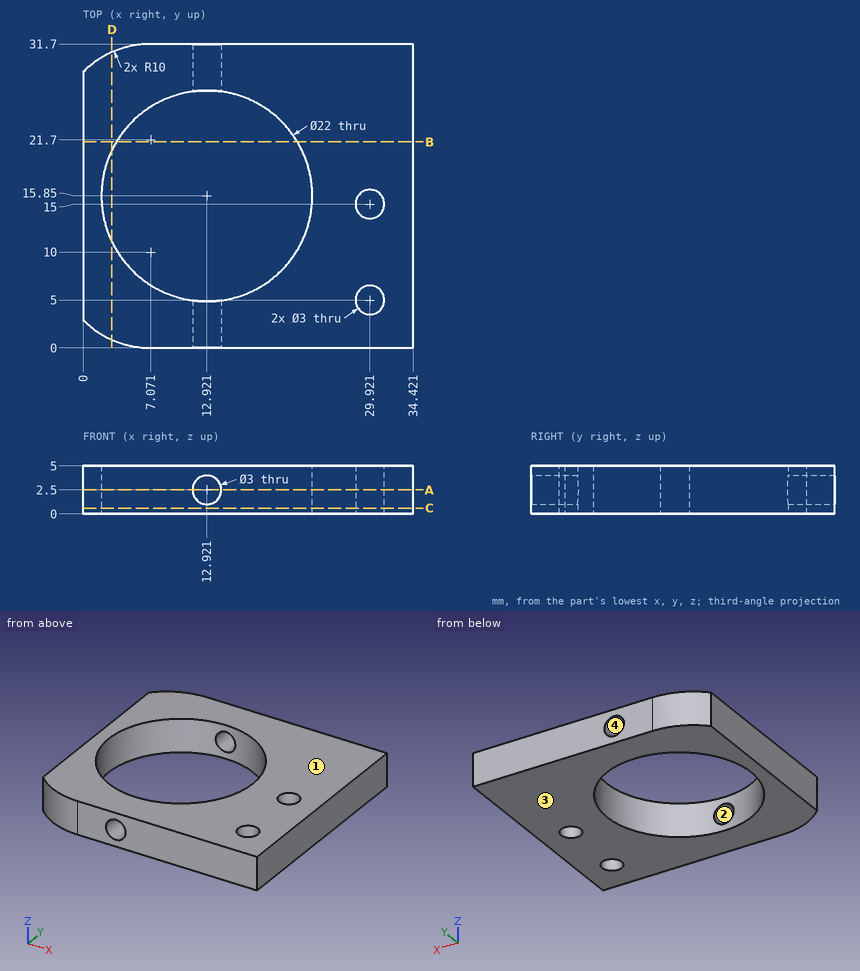
Input: dimensioned drawing with shaded views. Units: mm. Origin: part minimum x, y, z. Round coordinates to 2 decimals unless told otherwise and drop trailing zeros. Order: outer loops, then holes, each group sorted by start corner. A loop starts at its lowest first (then second) coordinate and runs counter-clockwise, first axis right, second up.
1. Cut plane D-D, the plane x = 3. Output: boundary loops of the cut face in (y, z), then the cut area to 3 significant figures.
The answers:
outline: (0.87, 0) - (11.1, 0) - (11.1, 5) - (0.87, 5) - close; (20.6, 0) - (30.83, 0) - (30.83, 5) - (20.6, 5) - close
area: 102 mm2
2. Cut plane A-A, the plane z = 2.5. Output: boundary loops of the cut face in (x, y), then the cut area to 3 significant figures.
The answers:
outline: (0, 2.93) arc R10 ccw to (7.07, 0) - (11.42, 0) - (11.42, 4.95) arc R11 cw to (11.42, 26.75) - (11.42, 31.7) - (7.07, 31.7) arc R10 ccw to (0, 28.77) - close; (14.42, 0) - (34.42, 0) - (34.42, 31.7) - (14.42, 31.7) - (14.42, 26.75) arc R11 cw to (14.42, 4.95) - close; hole circle Ø3 at (29.92, 5); hole circle Ø3 at (29.92, 15)
area: 655 mm2
3. Mould query, pull axis Z, two halves, no side actions, for the marked faces 1, 2, 3 and 4. Classes: released by +Z, released by -Z, zero draft, split by the parting line, or undercut.
The answers:
face 1: released by +Z
face 2: undercut
face 3: released by -Z
face 4: undercut
4. Cut plane B-B, the plane y = 21.5. Output: boundary loops of the cut face in (x, z).
The answers:
outline: (0, 0) - (3.48, 0) - (3.48, 5) - (0, 5) - close; (22.36, 0) - (34.42, 0) - (34.42, 5) - (22.36, 5) - close
5. Cut plane C-C, the plane z = 0.6. Output: boundary loops of the cut face in (x, y).
The answers:
outline: (0, 2.93) arc R10 ccw to (7.07, 0) - (34.42, 0) - (34.42, 31.7) - (7.07, 31.7) arc R10 ccw to (0, 28.77) - close; hole circle Ø22 at (12.92, 15.85); hole circle Ø3 at (29.92, 5); hole circle Ø3 at (29.92, 15)
6. Material intervals for line 1 (Y direction, x = 9, z = 3.3); line 2 (Y direction, x = 8, z = 1.4); line 3 (X direction, y = 2, z = 2.5), sorted ascending.
The answers:
line 1: y = 0 to 5.57, 26.13 to 31.7
line 2: y = 0 to 6.01, 25.69 to 31.7
line 3: x = 1.07 to 11.42, 14.42 to 34.42
